Could you check a few things on this model? Use its own coordinates, in mm. A direction names the side the tool comes from. Round coordinates to 2 decimals unless told otherwise and drop trailing zeros. Loops run counter-clockwise (first coordinate to the right, second up) from the corner with the lowest first, then second, coordinate; pieces in that order, holes last. Notation, with made-up numbers: (-17.5, 81) -> (38.5, 81) arc R21 ccw to (38.5, 114) -> close; hole circle Ø3 at (73, -21.75). An arc over 180 degrees is marked (long way). Put each result on its own line as item: value. Start each with the question number.
1. I'm going to push flat-ended pins straight in: P1, Ø6.5, axis at x = 3, y = -13.5, coming from the +Z side; P2, Ø1, axis at y = 5, z = 5.5, coming from the -X side. Where does each tip first touch, or does it pass through?
2. If we mould it in two halves opening along Y, with no side actions, what happens to faces 1 (the cylindrical face through (-1.34, 2.61, 3.94)), 2 (the flat face through (-6, -27, 4)), 3 (the flat face through (-4.977, 5.175, 3.944)), 4 (the flat face through (2, 19, 4))? For each: pulls with the +Y half, pulls with the -Y half, needs draft (parallel to the pull), parting line crosses it, or undercut.
3. Imagine slicing it at D-D, the plane z = 3. Count the separate pieces of the cut face and the enclosed holes in it, and give its area (3 significant figures).
4. Imagine slicing it at A-A, the plane y = -23.5. Please give me the cut outline in (x, z) (3 decimals), and give its area (3 significant figures).
5. Imagine slicing it at C-C, the plane y = 0.5. Please give me the cut outline in (x, z).
6. Which directions (+Z, -Z, +X, -X, +Y, -Y) give clear straight access to the entire face, cutting with the end or side of a thin tool? Please do faces 5 (the flat face through (0, -12, 1.999)), 6 (the cylindrical face through (3.99, -21.864, 3.944)), 7 (the flat face through (-2, 19, 4)).
7. I need wall thicknesses on line 1 (Y direction, x = 0, z = 5.75); line 2 (X direction, y = -25, z = 3.5); line 3 (X direction, y = 2, z = 6.25). Which ranges of each line are inside material? Lowest first, please. Write a range as [from, to].
8. Imagine slicing it at B-B, the plane x = 0. Please give me the cut outline in (y, z).
```python
from build123d import *

# Parameters (mm, degrees)
ESQUISSE1_W                             = 13
ESQUISSE1_H                             = 55
BOSS_EXTRU_1_DEPTH                      = 8
TROUS_DE_CENTRAGE_5_0MMTRANSITIONAL_1_D = 5
ESQUISSE4_W                             = 4.5
ESQUISSE4_H                             = 20
ENL_V_MAT_EXTRU_1_DEPTH                 = 30.368350311
CONG_1_R                                = 2
CHANFREIN1_SIZE                         = 1
TROU_TARAUD_M41_D                       = 3.3
CHANFREIN2_START                        = -1
CHANFREIN2_DEPTH                        = 10
ESQUISSE9_W                             = 8
ESQUISSE9_H                             = 8
ENL_V_MAT_EXTRU_2_DEPTH                 = 30.874738493
ESQUISSE10_W                            = 4
ESQUISSE10_H                            = 8
BOSS_EXTRU_2_DEPTH                      = 7
CHANFREIN3_SIZE                         = 1
BOSS_EXTRU_3_START                      = -8
BOSS_EXTRU_3_DEPTH                      = 8
CONG_2_R                                = 8
ESQUISSE12_W                            = 6.001123603
ESQUISSE12_H                            = 15.09853113
ENL_V_MAT_EXTRU_3_DEPTH                 = 32.452345059


with BuildPart() as part:
    # Esquisse1 → Boss.-Extru.1 (new body)
    with BuildSketch(Plane.XY):
        Rectangle(ESQUISSE1_W, ESQUISSE1_H)
    extrude(amount=BOSS_EXTRU_1_DEPTH)

    # Trous de centrage Ø5.0mmTransitional 1 (through all)
    with Locations(Plane.XY.offset(8)):
        with Locations((0, 0.5)):
            Hole(TROUS_DE_CENTRAGE_5_0MMTRANSITIONAL_1_D / 2)

    # Esquisse4 → Enlèv. mat.-Extru.1 (cut, through all)
    with BuildSketch(Plane.XY.offset(8)):
        with Locations((4.25, 17.5)):
            Rectangle(ESQUISSE4_W, ESQUISSE4_H)
        with Locations((-4.25, 17.5)):
            Rectangle(ESQUISSE4_W, ESQUISSE4_H)
    extrude(amount=-ENL_V_MAT_EXTRU_1_DEPTH, mode=Mode.SUBTRACT)

    # Congé1
    cong_1_edges = [part.edges().sort_by_distance(p)[0] for p in [
        (2, 7.5, 4),
        (-2, 7.5, 4),
    ]]
    fillet(cong_1_edges, radius=CONG_1_R)

    # Chanfrein1
    chanfrein1_edges = [part.edges().sort_by_distance(p)[0] for p in [
        (6.5, -27.5, 4),
        (-6.5, -27.5, 4),
    ]]
    chamfer(chanfrein1_edges, length=CHANFREIN1_SIZE)

    # Trou taraudé M41 (through all)
    with Locations(Plane.XY.offset(8)):
        with Locations((-3.775, -23.5), (3.775, -23.5)):
            Hole(TROU_TARAUD_M41_D / 2)

    # Chanfrein2: read off the stored shape, not the designer's step
    # Chanfrein2 outline → Chanfrein2 (cut)
    with BuildSketch(Plane.XY.offset(CHANFREIN2_START)):
        with BuildLine():
            Line((3.285714286, 7.631900453), (6.5, 2.961651585))
            Line((6.5, 2.961651585), (6.5, 7.5))
            Line((6.5, 7.5), (4, 7.5))
            ThreePointArc((4, 7.5), (3.636818981, 7.533251529), (3.285714286, 7.631900453))
        make_face()
        with BuildLine():
            Line((-6.5, 2.961651585), (-3.285714286, 7.631900453))
            ThreePointArc((-3.285714286, 7.631900453), (-3.636818981, 7.533251529), (-4, 7.5))
            Line((-4, 7.5), (-6.5, 7.5))
            Line((-6.5, 7.5), (-6.5, 2.961651585))
        make_face()
    extrude(amount=CHANFREIN2_DEPTH, mode=Mode.SUBTRACT)

    # Esquisse9 → Enlèv. mat.-Extru.2 (cut, through all)
    with BuildSketch(Plane.ZY.offset(2)):
        with Locations((4, 23.5)):
            Rectangle(ESQUISSE9_W, ESQUISSE9_H)
    extrude(amount=-ENL_V_MAT_EXTRU_2_DEPTH, mode=Mode.SUBTRACT)

    # Esquisse10 → Boss.-Extru.2 (add)
    with BuildSketch(Plane(origin=(0, 19.5, 0), x_dir=(1, 0, 0), z_dir=(0, 1, 0))):
        with Locations((0, -4)):
            Rectangle(ESQUISSE10_W, ESQUISSE10_H)
    extrude(amount=BOSS_EXTRU_2_DEPTH)

    # Chanfrein3
    chanfrein3_edges = [part.edges().sort_by_distance(p)[0] for p in [
        (0, 26.5, 0),
        (0, 26.5, 8),
    ]]
    chamfer(chanfrein3_edges, length=CHANFREIN3_SIZE)

    # Esquisse11 → Boss.-Extru.3 (add)
    with BuildSketch(Plane.XY.offset(8).offset(BOSS_EXTRU_3_START)):
        with BuildLine():
            Line((-3.285714286, 7.631900453), (-2, 9.5))
            ThreePointArc((-2, 9.5), (-2.352491058, 8.366106581), (-3.285714286, 7.631900453))
        make_face()
        with BuildLine():
            Line((3.285714286, 7.631900453), (2, 9.5))
            ThreePointArc((2, 9.5), (2.352491058, 8.366106581), (3.285714286, 7.631900453))
        make_face()
    extrude(amount=BOSS_EXTRU_3_DEPTH)

    # Congé2
    cong_2_edges = [part.edges().sort_by_distance(p)[0] for p in [
        (-2, 9.5, 4),
        (2, 9.5, 4),
    ]]
    fillet(cong_2_edges, radius=CONG_2_R)

    # Esquisse12 → Enlèv. mat.-Extru.3 (cut, through all)
    with BuildSketch(Plane(origin=(6.5, 0, 0), x_dir=(0, 0, -1), z_dir=(1, 0, 0))):
        with Locations((-4.999438199, -11.898438915)):
            Rectangle(ESQUISSE12_W, ESQUISSE12_H)
    extrude(amount=-ENL_V_MAT_EXTRU_3_DEPTH, mode=Mode.SUBTRACT)


solid = part.part
```
Entries:
1. P1: z = 2
1. P2: x = -5.44
2. face 1: undercut
2. face 2: pulls with the -Y half
2. face 3: pulls with the +Y half
2. face 4: needs draft
3. separate pieces: 2
3. enclosed holes: 3
3. area: 287 mm^2
4. outline: (-6.5, 0) -> (-5.425, 0) -> (-5.425, 8) -> (-6.5, 8) -> close; (-2.125, 0) -> (2.125, 0) -> (2.125, 8) -> (-2.125, 8) -> close; (5.425, 0) -> (6.5, 0) -> (6.5, 8) -> (5.425, 8) -> close
4. area: 51.2 mm^2
5. outline: (-6.5, 0) -> (-2.5, 0) -> (-2.5, 8) -> (-6.5, 8) -> close; (2.5, 0) -> (6.5, 0) -> (6.5, 8) -> (2.5, 8) -> close
6. face 5: +Z, +X, -X
6. face 6: +Z, -Z
6. face 7: +Z, -Z, -X, +Y
7. line 1: [-27.5, -19.45], [-4.35, -2], [3, 26.5]
7. line 2: [-6.5, -4.46], [-3.09, 3.09], [4.46, 6.5]
7. line 3: [-6.5, -2], [2, 6.5]
8. outline: (-27.5, 0) -> (-2, 0) -> (-2, 8) -> (-4.35, 8) -> (-4.35, 2) -> (-19.45, 2) -> (-19.45, 8) -> (-27.5, 8) -> close; (3, 0) -> (25.5, 0) -> (26.5, 1) -> (26.5, 7) -> (25.5, 8) -> (3, 8) -> close
